Could you check a few things on this model? Use its own coordinates, in mm. Face numbers are marked on the shaded views. A direction names the side the tool comes from. Coordinates: 2 decimals unless noted, no trailing zeros. Order: outer loops, then holes, each group sorted by start corner. A loop starts at its lowest first (then second) coordinate and runs counter-clockwise, first axis right, second up. Notation, with made-up numbers: (-38.75, 64.25) - (1.25, 64.25) arc R22 cw to (1.25, 83.25) - close; hole circle Ø9 at (-18.5, -26.75). An arc over 180 degrees is marked (long way). One line per item, written item: value.
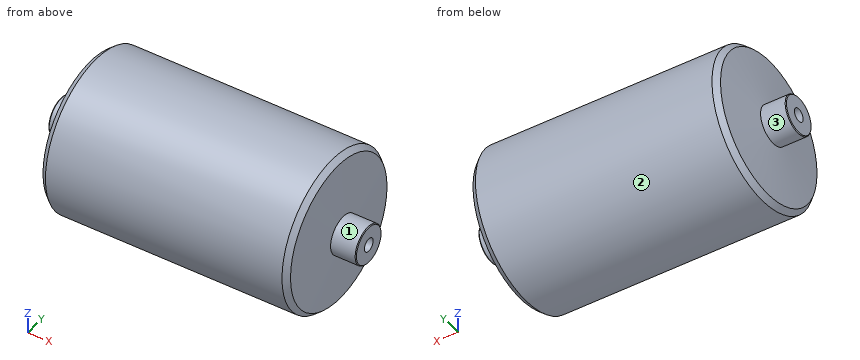
from build123d import *

# Parameters (mm, degrees)
TALADRO_ROSCADO_M102_D     = 8.5
TALADRO_ROSCADO_M102_DEPTH = 56.446342369
TALADRO_ROSCADO_M102_TIP   = 2.553657631


with BuildPart() as part:
    # Croquis1 → Revolución1 (revolve)
    with BuildSketch(Plane.XY):
        Polygon((0, 0), (0, 12), (0.5, 12.5), (16.5, 12.5), (19.519357654, 47.011415906), (23.081013485, 50), (176.918986515, 50), (180.480642346, 47.011415906), (183.5, 12.5), (199.5, 12.5), (200, 12), (200, 0), align=None)
    revolve(axis=Axis((200, 0, 0), (-1, 0, 0)))

    # Croquis4 → Taladro roscado M101 (revolve, cut)
    with BuildSketch(Plane(origin=(200, 0, 0), x_dir=(0, 0, -1), z_dir=(0, 1, 0))):
        Polygon((0, 0), (0, 59), (4.25, 56.446342369), (4.25, 0), align=None)
    revolve(axis=Axis((206.35, 0, 0), (-1, 0, 0)), mode=Mode.SUBTRACT)

    # Taladro roscado M102
    with Locations(Plane(origin=(0, 0, 0), x_dir=(0, -1, 0), z_dir=(-1, 0, 0))):
        with Locations((0, 0)):
            Hole(TALADRO_ROSCADO_M102_D / 2, depth=TALADRO_ROSCADO_M102_DEPTH)
            with Locations((0, 0, -(TALADRO_ROSCADO_M102_DEPTH + TALADRO_ROSCADO_M102_TIP / 2))):  # 118° drill point
                Cone(0, TALADRO_ROSCADO_M102_D / 2, TALADRO_ROSCADO_M102_TIP, mode=Mode.SUBTRACT)


solid = part.part
Item 1: For the marked faces 1, 2 and 3, which set-ups out of +Z, -Z, +X, -X, +Y, -Y let a thin tool reach every point of the face, with its end or its side?
Conclusion:
face 1: +X
face 2: +X, -X
face 3: -X
Item 2: I want a section at A-A on x = 51. Please give me the cut outline in (y, z).
Conclusion:
outline: circle Ø100 at (0, 0); hole circle Ø8.5 at (0, 0)
Item 3: If I drill on probe 1 along Z at (x, y) = (40, 0); probe 2 along Z at (x, y) = (191.5, -5), over which ranges is the centre line in solid material (lowest first)?
Conclusion:
probe 1: -50 to -4.25, 4.25 to 50
probe 2: -11.46 to 11.46
Item 4: I want a section at B-B on x = 129. Please give me the cut outline in (y, z).
Conclusion:
outline: circle Ø100 at (0, 0)
Item 5: I'm going to push flat-ended pins straight in: pin 1 Ø8 at (x, z) = (54, -4.5) entering from -Y; pin 2 Ø1.5 at (x, y) = (56, 38) entering from +Z; pin 3 Ø6 at (y, z) = (24, -37) entering from -X; pin 4 Ø12 at (y, z) = (3.5, -8) entering from -X. Where does each tip first touch, or does it pass through?
Conclusion:
pin 1: y = -50
pin 2: z = 33.35
pin 3: x = 19
pin 4: x = 0
